Source: CAD feature listing. Evaluate the final solid. Frame: model axes, mm. A direction names the side the tool comes from. Round coordinates to 2 decimals unless told otherwise and drop trailing zeros. Order: outer loops, then holes, each group sorted by start corner. A loop starts at its lowest first (then second) coordinate and runs counter-clockwise, first axis right, second up. Notation, with made-up numbers: (-2.75, -14) - (35.25, -14) arc R24 cw to (35.25, 21) - close; hole circle Ø8 at (-15, 79.25). An arc over 180 degrees is marked (long way). Put each result on its own line as item: value. Start each with the question number.
1) Access query for faces 4 (the face through (9.25, -7, 123)), 5 (the face through (-9.25, -7, 123)), 6 (the face through (-0.29, 17.36, 123.25)), 7 (the face through (5.81, -0.7, 123.25)). Directions: +Z, -Z, +X, -X, +Y, -Y. A direction counts if a zero-diameter tool reaches every point of the face in a straight line with its end or side. Return the directions, or none.
2) Line query: probe 1 along Z at (x, y) = (15, -11.55); probe 2 along X at (y, z) = (-14, 150); probe 3 along Y at (x, z) = (10, 75). Output: solid intervals per line, ascending. Write a range as [from, to].
3) Section C-C on z = 211.5. Output: boundary loops of the cut face in (x, y), then the cut area to 3 significant figures.
4) Mould query, pull axis X, two halves, no side actions, for faces 1 (the face through (0, -3, 0)), 2 (the face through (14.17, -13.1, 147.38)), 3 (the face through (-5.81, -0.7, 123.25)). Classes: +X half, -X half, draft (parallel to the pull), parting line (faces both ways), or undercut.
5) Contact query for flat-ended pins moving along their axis: P1, Ø9, axis at x = -15, z = 225, coming from the -Y side; P2, Ø1.5, axis at y = 13, z = 44.5, coming from the -X side; P3, Ø9, axis at x = 15, z = 75, coming from the +Y side; P4, Ø0.8, axis at x = -8.5, z = 90.5, coming from the +Y side. Output: stop coordinate, or through.
6) Section B-B on z = 75. Output: boundary loops of the cut face in (x, y), then the cut area to 3 significant figures.
7) Section D-D on y = 0. Output: boundary loops of the cut face in (x, z).
8) Section A-A on x = -15. Output: boundary loops of the cut face in (y, z).
Autodesk Inventor part; units mm, degrees
ref_plane "YZ Plane" through (0, 0, 0) normal (1, 0, 0) x (0, 1, 0)
ref_plane "XZ Plane" through (0, 0, 0) normal (0, 1, 0) x (-1, 0, 0)
ref_plane "XY Plane" through (0, 0, 0) normal (0, 0, 1) x (1, 0, 0)
sketch "Esboço1" plane through (0, 0, 0) normal (0, 0, 1) x (1, 0, 0)
  arc A0 (4, 2.4377) -> (-4, 2.4377) centre (0, 9.3659) ccw
  line L0 (9.25, -3.9341) -> (9.25, -10.6341)
  line L1 (-9.25, -10.6341) -> (-9.25, -3.9341)
  line L2 (4, -15.6341) -> (-4, -15.6341)
  line L3 (20, -15.6341) -> (-20, -15.6341)
  line L4 (-20, -15.6341) -> (-20, -10.6341)
  line L5 (20, -10.6341) -> (20, -15.6341)
  line L6 (7.6788, -3.9341) -> (9.25, -3.9341)
  line L7 (-9.25, -3.9341) -> (-7.6788, -3.9341)
  line L8 (9.25, -10.6341) -> (20, -10.6341)
  line L9 (-20, -10.6341) -> (-9.25, -10.6341)
  line L10 (-4, 2.4377) -> (-7.6788, -3.9341)
  line L11 (-17.4151, -20.798) -> (-22.4188, -29.4646)
  line L12 (17.4151, -20.798) -> (23.6527, -31.6017)
  line L13 (9.25, -15.6341) -> (4, -15.6341)
  line L14 (0, -15.6341) -> (-9.25, -15.6341)
  line L15 (4, 2.4377) -> (7.6788, -3.9341)
  dimension "d6" = 16
  dimension "d7" = 25
  dimension "d8" = 18.5
  dimension "d9" = 11.7
  dimension "d10" = 8
  dimension "d13" = 5
  dimension "d14" = 40
extrude "Extrusão1" add sketch "Esboço1" along normal blind 250
sketch "Esboço3" plane through (-20, -15.6341, 0) normal (0, -1, 0) x (1, 0, 0)
  line L0 (0, 250) -> (40, 250) construction
  line L1 (20, 250) -> (20, 0) construction
  line L2 (20, 225) -> (5, 225) construction
  line L3 (5, 225) -> (20, 225) construction
  line L4 (20, 225) -> (35, 225) construction
  circle A0 centre (5, 225) radius 2.75
  circle A1 centre (35, 225) radius 2.75
  line L5 (40, 0) -> (0, 0) construction
  line L6 (35, 250) -> (35, 0) construction
  line L7 (5, 250) -> (5, 0) construction
  circle A2 centre (35, 150) radius 2.75
  circle A3 centre (35, 75) radius 2.75
  circle A4 centre (35, 0) radius 2.75
  circle A5 centre (5, 150) radius 2.75
  circle A6 centre (5, 75) radius 2.75
  circle A7 centre (5, 0) radius 2.75
  dimension "d18" = 15
  dimension "d19" = 15
  dimension "d20" = 5.5
  dimension "d21" = 5.5
  dimension "d22" = 25
  dimension "d37" = 75
  dimension "d44" = 75
hole "Furo2" at (15, -15.6341, 225) at (-15, -15.6341, 225) at (-15, -15.6341, 150) at (15, -15.6341, 150) at (-15, -15.6341, 75) at (15, -15.6341, 75) at (15, -15.6341, 0) at (-15, -15.6341, 0) direction (0, 1, 0) diameter 5.5 end through all
properties part number "SBR16_200MM"
Answer sheet:
1. face 4: +Z, -Z, +X, +Y
1. face 5: +Z, -Z, -X, +Y
1. face 6: +Z, -Z
1. face 7: +Z, -Z, +X
2. probe 1: [2.75, 72.25], [77.75, 147.25], [152.75, 222.25], [227.75, 250]
2. probe 2: [-20, -17.75], [-12.25, 12.25], [17.75, 20]
2. probe 3: [-15.63, -10.63]
3. outline: (-20, -15.63) - (20, -15.63) - (20, -10.63) - (9.25, -10.63) - (9.25, -3.93) - (7.68, -3.93) - (4, 2.44) arc R8 ccw (long way) to (-4, 2.44) - (-7.68, -3.93) - (-9.25, -3.93) - (-9.25, -10.63) - (-20, -10.63) - close
3. area: 594 mm^2
4. face 1: draft
4. face 2: undercut
4. face 3: -X half
5. P1: y = -15.63
5. P2: x = -7.46
5. P3: y = -10.63
5. P4: y = -3.93
6. outline: (-20, -15.63) - (-17.75, -15.63) - (-17.75, -10.63) - (-20, -10.63) - close; (-12.25, -15.63) - (12.25, -15.63) - (12.25, -10.63) - (9.25, -10.63) - (9.25, -3.93) - (7.68, -3.93) - (4, 2.44) arc R8 ccw (long way) to (-4, 2.44) - (-7.68, -3.93) - (-9.25, -3.93) - (-9.25, -10.63) - (-12.25, -10.63) - close; (17.75, -15.63) - (20, -15.63) - (20, -10.63) - (17.75, -10.63) - close
6. area: 539 mm^2
7. outline: (-5.41, 0) - (5.41, 0) - (5.41, 250) - (-5.41, 250) - close
8. outline: (-15.63, 2.75) - (-10.63, 2.75) - (-10.63, 72.25) - (-15.63, 72.25) - close; (-15.63, 77.75) - (-10.63, 77.75) - (-10.63, 147.25) - (-15.63, 147.25) - close; (-15.63, 152.75) - (-10.63, 152.75) - (-10.63, 222.25) - (-15.63, 222.25) - close; (-15.63, 227.75) - (-10.63, 227.75) - (-10.63, 250) - (-15.63, 250) - close
